Read the model definition and answer for the solid it produces. Units are mm, in the model's axes. Give positions to 0.01 mm unless a question says otherwise; leave off trailing zeros. Loops run counter-clockwise (first coordinate to the right, second up) from the corner with the lowest first, then second, coordinate; pieces in that order, holes last.
(1) Find section C-C, the plane z = 4.15. State how many separate pieces and enclosed holes the cut face has, then the cut area to 3 significant figures.
(2) Find section A-A, the plane y = 0. Write down the section's boundary in (x, z) (3 decimals).
(3) Determine the mould class of faces 1 (the face through (-55, -1, 2)), 2 (the face through (17.92, -41.6, 2.54)) for opening direction Y: pulls with the +Y half, pulls with the -Y half, needs draft (parallel to the pull), parting line crosses it, or undercut.
(4) Straight lines are drawn through the part: probe 1 along Y at (x, z) = (40, 2.5) (3 decimals); probe 2 along X at (y, z) = (-41, 3.5); probe 3 along X at (y, z) = (38.5, 1.1). For each, find the intervals that lie inside material, in ascending order.
```python
from build123d import *

# Parameters (mm, degrees)
SKETCH_W     = 110
SKETCH_H     = 110
PAD_DEPTH    = 5
SKETCH001_R  = 2.625
POCKET_DEPTH = 5


with BuildPart() as part:
    # Sketch → Pad (new body)
    with BuildSketch(Plane.XY):
        Rectangle(SKETCH_W, SKETCH_H)
    extrude(amount=PAD_DEPTH)

    # Sketch001 (on Face6 of Pad) → Pocket (cut)
    with BuildSketch(Plane.XY.offset(5)):
        Circle(SKETCH001_R)
        with Locations((20, 0)):
            Circle(SKETCH001_R)
        with Locations((40, 0)):
            Circle(SKETCH001_R)
        with Locations((-20, 0)):
            Circle(SKETCH001_R)
        with Locations((-40, 0)):
            Circle(SKETCH001_R)
        with Locations((-40, 20)):
            Circle(SKETCH001_R)
        with Locations((-40, 40)):
            Circle(SKETCH001_R)
        with Locations((-20, 20)):
            Circle(SKETCH001_R)
        with Locations((-20, 40)):
            Circle(SKETCH001_R)
        with Locations((0, 20)):
            Circle(SKETCH001_R)
        with Locations((0, 40)):
            Circle(SKETCH001_R)
        with Locations((20, 20)):
            Circle(SKETCH001_R)
        with Locations((20, 40)):
            Circle(SKETCH001_R)
        with Locations((40, 20)):
            Circle(SKETCH001_R)
        with Locations((40, 40)):
            Circle(SKETCH001_R)
        with Locations((0, -20)):
            Circle(SKETCH001_R)
        with Locations((0, -40)):
            Circle(SKETCH001_R)
        with Locations((20, -20)):
            Circle(SKETCH001_R)
        with Locations((20, -40)):
            Circle(SKETCH001_R)
        with Locations((40, -20)):
            Circle(SKETCH001_R)
        with Locations((40, -40)):
            Circle(SKETCH001_R)
        with Locations((-20, -40)):
            Circle(SKETCH001_R)
        with Locations((-20, -20)):
            Circle(SKETCH001_R)
        with Locations((-40, -20)):
            Circle(SKETCH001_R)
        with Locations((-40, -40)):
            Circle(SKETCH001_R)
    extrude(amount=-POCKET_DEPTH, mode=Mode.SUBTRACT)


solid = part.part
```
Entries:
1. separate pieces: 1
1. enclosed holes: 25
1. area: 11,600 mm2
2. outline: (-55, 0) - (-42.625, 0) - (-42.625, 5) - (-55, 5) - close; (-37.375, 0) - (-22.625, 0) - (-22.625, 5) - (-37.375, 5) - close; (-17.375, 0) - (-2.625, 0) - (-2.625, 5) - (-17.375, 5) - close; (2.625, 0) - (17.375, 0) - (17.375, 5) - (2.625, 5) - close; (22.625, 0) - (37.375, 0) - (37.375, 5) - (22.625, 5) - close; (42.625, 0) - (55, 0) - (55, 5) - (42.625, 5) - close
3. face 1: needs draft
3. face 2: undercut
4. probe 1: y = -55 to -42.625, -37.375 to -22.625, -17.375 to -2.625, 2.625 to 17.375, 22.625 to 37.375, 42.625 to 55
4. probe 2: x = -55 to -42.43, -37.57 to -22.43, -17.57 to -2.43, 2.43 to 17.57, 22.43 to 37.57, 42.43 to 55
4. probe 3: x = -55 to -42.15, -37.85 to -22.15, -17.85 to -2.15, 2.15 to 17.85, 22.15 to 37.85, 42.15 to 55
